Can you work these out from the model? Positions are in its coordinate system, mm. A direction names the side the tool comes from. Coordinates: 2 decimals unless noted, no trailing zeros. Loops run counter-clockwise (first coordinate to the right, second up) from the corner with the lowest first, then second, coordinate; pieces in that order, holes last. Notation, with made-up numbers: (55.5, 25.5) -> (76.5, 25.5) arc R10 cw to (76.5, 39.5) -> close; hole circle Ø6 at (70.5, 44). An arc over 180 degrees is marked (long way). Use one line per item in the form item = value. Start each with the question number.
(1) On a 3-axis mill with a long thin cutter (end or side, diameter ignored), from which of +Z, -Z, +X, -X, +Y, -Y can I reach the whole of each face in a straight line? I mean faces 1 (the flat face through (60.35, 49.58, -49.3)), 2 (the flat face through (85.7, 59.72, -49.3)), 3 (the flat face through (95, 34, -70)). Say none if no direction works.
(2) I'm going to push flat-ended pins straight in: pin 1 (6 mm diameter, centred on x = 64.5, y = 63, fed in from +Z); pin 2 (1 mm diameter, centred on y = 54, z = -17.5, fed in from -X); pin 3 (12 mm diameter, centred on y = 50.5, z = -51.5, fed in from +X). Where does each tip first touch, or does it pass through?
(3) Imagine slicing it at D-D (z = -33). List the corners of the cut face in (x, y) for me.
(4) Thinking about a two-plate mould opening in Z: for faces 4 (the flat face through (50, 57, -38)), 5 (the flat face through (95, 26, -30)), 6 (the flat face through (49, 32, 0)), 7 (the flat face through (90, 27, -50)), which applies, released by +Z, released by -Z, zero draft, split by the parting line, or undercut?
(5) I need wall thicknesses on line 1 (X direction, y = 26, z = -6); line 2 (Z direction, x = 92.5, y = 30); line 3 (X direction, y = 22.5, z = -39). Which ranges of each line are inside material? Lowest first, please. Write a range as [from, to].
(6) Imagine slicing it at C-C (x = 85). List the corners of the cut face in (y, z) for me, plus the area to 3 significant figures.
(7) Imagine slicing it at A-A (z = -44). List the corners of the cut face in (x, y) for me.
(8) Imagine slicing it at B-B (y = 54.5). List the corners of the cut face in (x, z) for me.
```python
from build123d import *

# Parameters (mm, degrees)
SKETCH1_W               = 100
SKETCH1_H               = 80
BOSS_EXTRUDE1_DEPTH     = 100
CUT_EXTRUDE1_DEPTH      = 30
CUT_EXTRUDE2_DEPTH      = 50
CUT_EXTRUDE4_DEPTH      = 1
CUT_EXTRUDE4_DEPTH_BACK = 20
CUT_EXTRUDE4_START      = -30
CUT_EXTRUDE3_DEPTH      = 10


with BuildPart() as part:
    # Sketch1 → Boss-Extrude1 (new body)
    with BuildSketch(Plane.XY):
        with Locations((50, 40)):
            Rectangle(SKETCH1_W, SKETCH1_H)
    extrude(amount=-BOSS_EXTRUDE1_DEPTH)

    # Sketch3 → Cut-Extrude1 (cut)
    with BuildSketch(Plane.ZY):
        Polygon((0, 0), (-30, 80), (0, 80), align=None)
    extrude(amount=-CUT_EXTRUDE1_DEPTH, mode=Mode.SUBTRACT)

    # Sketch5 → Cut-Extrude2 (cut)
    with BuildSketch(Plane(origin=(100, 0, 0), x_dir=(0, 0, -1), z_dir=(1, 0, 0))):
        Polygon((0, 40), (100, 80), (0, 80), align=None)
    extrude(amount=-CUT_EXTRUDE2_DEPTH, mode=Mode.SUBTRACT)

    # Sketch8 → Cut-Extrude4 (cut, two sides: drawn at the far end of the back side and taken through both)
    with BuildSketch(Plane(origin=(100, 0, 0), x_dir=(0, 0, -1), z_dir=(1, 0, 0)).offset(CUT_EXTRUDE4_START - CUT_EXTRUDE4_DEPTH_BACK)):
        Polygon((0, 20), (100, 80), (0, 40), align=None)
    extrude(amount=CUT_EXTRUDE4_DEPTH + CUT_EXTRUDE4_DEPTH_BACK, mode=Mode.SUBTRACT)

    # Sketch7 → Cut-Extrude3 (cut)
    with BuildSketch(Plane(origin=(100, 0, 0), x_dir=(0, 0, -1), z_dir=(1, 0, 0))):
        Polygon((30, 52), (30, 0), (70, 0), (70, 68), align=None)
    extrude(amount=-CUT_EXTRUDE3_DEPTH, mode=Mode.SUBTRACT)


solid = part.part
```
Worked out:
q1.face_1 = +Z, +Y
q1.face_2 = +Z, +X, +Y
q1.face_3 = +X, +Y, -Y
q2.pin_1 = -66.67
q2.pin_2 = 30
q2.pin_3 = 90
q3.outline = (0, 0) -> (90, 0) -> (90, 53.2) -> (71, 53.2) -> (71, 39.8) -> (50, 39.8) -> (50, 80) -> (0, 80) -> close
q4.face_4 = zero draft
q4.face_5 = undercut
q4.face_6 = released by +Z
q4.face_7 = undercut
q5.line_1 = [30, 50], [71, 100]
q5.line_2 = [-100, -70], [-30, 0]
q5.line_3 = [0, 90]
q6.outline = (0, -100) -> (80, -100) -> (40, 0) -> (0, 0) -> close
q6.area = 6,000 mm2
q7.outline = (0, 0) -> (90, 0) -> (90, 57.6) -> (71, 57.6) -> (71, 46.4) -> (50, 46.4) -> (50, 80) -> (0, 80) -> close
q8.outline = (0, -100) -> (100, -100) -> (100, -70) -> (90, -70) -> (90, -36.25) -> (71, -36.25) -> (71, -57.5) -> (50, -57.5) -> (50, 0) -> (30, 0) -> (30, -20.44) -> (0, -20.44) -> close
